Read the model definition and answer for the solid it produces. Units are mm, in the model's axes. Give positions to 0.01 mm unless a question says otherwise; leave off trailing zeros. Order: outer loops, then holes, each group sorted by start corner. A loop starts at its lowest first (then second) coordinate and runs counter-clockwise, first axis right, second up. Notation, with made-up numbers: (-6, -22) - (30, -22) arc R32 cw to (30, 15) - close; hole circle Ø10 at (-39.75, -5.5). An arc over 180 degrees is marked (long way). Write item = value, one per line.
```python
from build123d import *

# Parameters (mm, degrees)
SKETCH_1_R      = 1.5
SKETCH_1_R_2    = 2
EXTRUDE_1_DEPTH = 2


with BuildPart() as part:
    # Эскиз1 → Бобышка-Вытянуть1 (new body)
    with BuildSketch(Plane(origin=(0, 0, 0), x_dir=(1, 0, 0), z_dir=(0, 1, 0))):
        with BuildLine():
            Line((12.374772085, -29.617278809), (12.374772085, 20.682721191))
            Line((12.374772085, 20.682721191), (9.374772085, 39.182721191))
            ThreePointArc((9.374772085, 39.182721191), (-2.625227915, 51.182721191), (-14.625227915, 39.182721191))
            Line((-14.625227915, 39.182721191), (-17.625227915, 20.682721191))
            Line((-17.625227915, 20.682721191), (-17.625227915, -29.617278809))
            Line((-17.625227915, -29.617278809), (-10.625227915, -29.617278809))
            Line((-10.625227915, -29.617278809), (5.374772085, -29.617278809))
            Line((5.374772085, -29.617278809), (12.374772085, -29.617278809))
        make_face()
        with Locations(Location((-13.625227915, -26.117278809, 0), (0, 0, 270))):
            Circle(SKETCH_1_R, mode=Mode.SUBTRACT)
        with Locations(Location((8.374772085, -26.117278809, 0), (0, 0, 270))):
            Circle(SKETCH_1_R, mode=Mode.SUBTRACT)
        with Locations(Location((-2.625227915, 39.182721191, 0), (0, 0, 270))):
            Circle(SKETCH_1_R_2, mode=Mode.SUBTRACT)
    extrude(amount=EXTRUDE_1_DEPTH)


solid = part.part
```
1. Section C-C (x = -8.25) is taken. Determine the outline of the cut face in (y, z), and give its area (3 significant figures).
Recorded:
outline = (0, -49.78) - (2, -49.78) - (2, 29.62) - (0, 29.62) - close
area = 159 mm^2
2. Section B-B (z = -23.5) is taken. Determine the outline of the cut face in (x, y).
Recorded:
outline = (-17.17, 0) - (11.92, 0) - (11.92, 2) - (-17.17, 2) - close
3. Section A-A (y = 1.2) is taken. Determine the outline of the cut face in (x, z).
Recorded:
outline = (-17.63, -20.68) - (-14.63, -39.18) arc R12 ccw to (9.37, -39.18) - (12.37, -20.68) - (12.37, 29.62) - (-17.63, 29.62) - close; hole circle Ø3 at (-13.63, 26.12); hole circle Ø4 at (-2.63, -39.18); hole circle Ø3 at (8.37, 26.12)
4. Straight lines are drawn through the part: L1, parallel to Z at x = 7.25, y = 1.15; L2, parallel to Z at x = -2.75, y = 1.35; L3, parallel to Z at x = 3.5, y = 1.5. For each, find the intervals that lie inside material, in ascending order. Write a range as [from, to].
Recorded:
L1 = [-46, 25.12], [27.11, 29.62]
L2 = [-51.18, -41.18], [-37.19, 29.62]
L3 = [-49.5, 29.62]
5. Determine the mould class of faces 1 (the face through (-2.54, 0.99, -41.18)), 2 (the face through (8.44, 0.99, 24.62)), 3 (the face through (-3, 1, 29.617)), 4 (the face through (-3, 2, -11)) for opening direction Z: +Z half, -Z half, draft (parallel to the pull), parting line (faces both ways), or undercut.
Recorded:
face_1 = undercut
face_2 = undercut
face_3 = +Z half
face_4 = draft
